The listing builds one solid part. Answer for the finished solid, in the listing's coordinates (mm). Face numbers are marked on the shaded views. A direction names the side the tool comes from. Give positions to 0.01 mm unless a question says otherwise; leave off trailing zeros. Order: outer loops, then holes, each group sorted by start corner. A loop starts at its lowest first (then second) coordinate and runs counter-clockwise, first axis right, second up. Notation, with made-up numbers: (-12, 22) - (16, 22) arc R35 cw to (16, 61) - close; hole circle Ø5 at (-11.75, -9). An arc over 180 degrees is marked (long way). Answer as CSV lines item,"result". Start each with the question number.
1. Section A-A on y = -7 is taken. Give the vertices of the cut face in (x, z), and give its area (3 significant figures).
2. Section C-C on z = 10 is taken. Give the vertices of the cut face in (x, y).
3. Determine the mould class of the marked faces 3, 4, 5 and 6 for opening direction X: +X half, -X half, draft (parallel to the pull), parting line (faces both ways), or undercut.
4. Section B-B on x = 22 is taken. Give the vertices of the cut face in (y, z), and give its area (3 significant figures).
5. Flat-ended cylindrical pins translate along their axes: pin 1 (0.9 mm diameter, centred on x = 57, y = -36, fed in from -Z); pin 2 (6 mm diameter, centred on y = -27, z = -21, fed in from +X); pin 3 (6 mm diameter, centred on y = -18, z = 15.5, fed in from -X); pin 4 (3 mm diameter, centred on x = 35.5, y = -38.5, fed in from +Z). Find the tip coordinate at first contact, or state that the pin passes through.
6. Which of the six approach directions +Z, -Z, +X, -X, +Y, -Y give full straight-line access (tool end or side, diameter ignored) to the marked faces 1 and 2?
7. Consider line 1 along Z through (x, y) = (-19, -67.5); line 2 along Z through (x, y) = (21, -51); line 3 along X through (y, z) = (-48, -28). Determine where each line is inside the solid, lowest interval first. Write a range as [from, to].
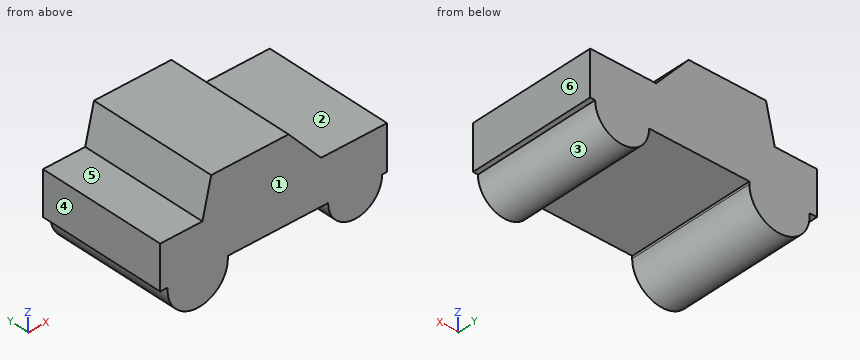
from build123d import *

# Parameters (mm, degrees)
F3_DEPTH = 76.2


with BuildPart() as f3:
    # F2 (on face) → F3 (new body)
    with BuildSketch(Plane.XZ):
        with BuildLine():
            ThreePointArc((23.432876, -18.704671), (39.391141, -2.962637), (55.349406, -18.704671))
            Line((55.349406, -18.704671), (58.282666, -18.704671))
            Line((58.282666, -18.704671), (58.282666, 7.556662))
            Line((58.282666, 7.556662), (19.231044, 7.556662))
            Line((19.231044, 7.556662), (0, 29.359408))
            Line((0, 29.359408), (-45.805167, 29.359408))
            Line((-45.805167, 29.359408), (-51.002167, 7.000253))
            Line((-51.002167, 7.000253), (-76.00525, 7.000253))
            Line((-76.00525, 7.000253), (-76.00525, -18.745113))
            Line((-76.00525, -18.745113), (-71.593166, -18.737061))
            ThreePointArc((-71.593166, -18.737061), (-53.815115, -2.368458), (-36.007295, -18.704671))
            Line((-36.007295, -18.704671), (23.432876, -18.704671))
        make_face()
        with BuildLine():
            Line((-53.844772, -18.704671), (-36.007295, -18.704671))
            ThreePointArc((-36.007295, -18.704671), (-53.815115, -2.368458), (-71.593166, -18.737061))
            Line((-71.593166, -18.737061), (-53.844772, -18.704671))
        make_face()
        with BuildLine():
            ThreePointArc((-35.942469, -20.224843), (-35.958683, -19.464066), (-36.007295, -18.704671))
            Line((-36.007295, -18.704671), (-53.844772, -18.704671))
            Line((-53.844772, -18.704671), (-71.593166, -18.737061))
            ThreePointArc((-71.593166, -18.737061), (-54.5434, -38.065707), (-35.942469, -20.224843))
        make_face()
        with BuildLine():
            ThreePointArc((23.432876, -18.704671), (39.282281, -34.881765), (55.350891, -18.922387))
            ThreePointArc((55.350891, -18.922387), (55.35052, -18.813527), (55.349406, -18.704671))
            Line((55.349406, -18.704671), (23.432876, -18.704671))
        make_face()
        with BuildLine():
            Line((23.432876, -18.704671), (55.349406, -18.704671))
            ThreePointArc((55.349406, -18.704671), (39.391141, -2.962637), (23.432876, -18.704671))
        make_face()
    extrude(amount=F3_DEPTH)


solid = f3.part
Checks:
1,outline,"(-76.01, -18.75) - (-71.59, -18.74) arc R17.86 ccw (long way) to (-35.94, -20.22) arc R17.86 ccw to (-36.01, -18.7) - (23.43, -18.7) arc R15.96 ccw (long way) to (55.35, -18.92) arc R15.95 ccw to (55.35, -18.7) - (58.28, -18.7) - (58.28, 7.56) - (19.23, 7.56) - (0, 29.36) - (-45.81, 29.36) - (-51, 7) - (-76.01, 7) - close"
1,area,"5,740 mm²"
2,outline,"(-50.3, -76.2) - (17.08, -76.2) - (17.08, 0) - (-50.3, 0) - close"
3,face 3,"undercut"
3,face 4,"-X half"
3,face 5,"draft"
3,face 6,"+X half"
4,outline,"(-76.2, -18.7) - (0, -18.7) - (0, 7.56) - (-76.2, 7.56) - close"
4,area,"2,000 mm²"
5,pin 1,"stops at z = -18.7"
5,pin 2,"stops at x = 58.28"
5,pin 3,"stops at x = -49.72"
5,pin 4,"stops at z = 7.56"
6,face 1,"+Z, -Z, +X, -X, -Y"
6,face 2,"+Z, +X, +Y, -Y"
7,line 1,"z = [-18.7, 29.36]"
7,line 2,"z = [-18.7, 7.56]"
7,line 3,"x = [-69.87, -37.72], [26.26, 52.52]"
